Source: CAD feature listing. Evaluate the final solid. Frame: model axes, mm. A direction names the side the tool comes from. Give positions to 0.01 mm unless a question says otherwise; leave off trailing zeros. Order: outer loops, then holes, each group sorted by start corner. A loop starts at its lowest first (then second) coordinate and runs counter-clockwise, first axis right, second up.
Autodesk Inventor part; units mm, degrees
ref_plane "YZ Plane" through (0, 0, 0) normal (1, 0, 0) x (0, 1, 0)
ref_plane "XZ Plane" through (0, 0, 0) normal (0, 1, 0) x (-1, 0, 0)
ref_plane "XY Plane" through (0, 0, 0) normal (0, 0, 1) x (1, 0, 0)
sketch "Sketch1" plane through (0, 0, 0) normal (0, 0, 1) x (1, 0, 0)
  circle A0 centre (0, 0) radius 6.35
  dimension "d0" = 12.7
extrude "Extrusion1" add sketch "Sketch1" along normal blind 5.08 and the other way blind 16.02
sketch "Sketch4" plane through (0, 0, 0) normal (0, 0, 1) x (1, 0, 0)
  circle A0 centre (0, 0) radius 12.065
  dimension "d9" = 24.13
extrude "Extrusion3" add sketch "Sketch4" against normal blind 1.02
sketch "Sketch5" plane through (0, 0, 5.08) normal (0, 0, 1) x (1, 0, 0)
  circle A0 centre (0, 0) radius 6.35
  circle A1 centre (0, 0) radius 2.415
  dimension "d12" = 4.83
extrude "Extrusion4" add sketch "Sketch5" along normal blind 6.86 contours A1
sketch "Sketch6" plane through (0, 0, 0) normal (0, 0, 1) x (1, 0, 0)
  circle A0 centre (0, 0) radius 6.35
  circle A1 centre (0, 9.21) radius 1.64
  circle A2 centre (0, 0) radius 9.21 construction
  line L0 (0, 0) -> (0, 14.2117) construction
  dimension "d15" = 18.42
  dimension "d16" = 3.28
extrude "Extrusion5" cut sketch "Sketch6" against normal through all contours A1
pattern_circular "Circular Pattern1" count 3 over 360 about axis through (0, 0, -10) along (0, 0, 1) of "Extrusion5"
properties part number "Slip_Ring"
1) Section query C-C, the plane y = 0. Return the cut outline in (x, z) (3 decimals).
Report:
outline: (-12.065, -1.02) - (-6.35, -1.02) - (-6.35, -16.02) - (6.35, -16.02) - (6.35, -1.02) - (12.065, -1.02) - (12.065, 0) - (6.35, 0) - (6.35, 5.08) - (2.415, 5.08) - (2.415, 11.94) - (-2.415, 11.94) - (-2.415, 5.08) - (-6.35, 5.08) - (-6.35, 0) - (-12.065, 0) - close
2) Material intervals for L1, parallel to Y at x = 0, z = -0.6 (3 decimals); L2, parallel to Z at x = 4.25, y = -5; L3, parallel to Z at x = -0.75, y = 6.25, sorted ascending.
Report:
L1: y = -12.065 to 7.57, 10.85 to 12.065
L2: z = -1.02 to 0
L3: z = -16.02 to 5.08
3) Pin query (flat end, axial travel): pin 1 (10 mm diameter, centred on y = 0.5, z = 7.5, fed in from +X); pin 2 (8 mm diameter, centred on y = 1.5, z = 8.5, fed in from -X); pin 3 (10 mm diameter, centred on y = -6.5, z = 0.5, fed in from -X). Return the tip coordinate at first contact, or that it passes through.
Report:
pin 1: stops at x = 6.35
pin 2: stops at x = -6.35
pin 3: stops at x = -11.97
4) Section query A-A, the plane x = 0. Return the cut outline in (y, z) (3 decimals), and give its area (3 significant figures).
Report:
outline: (-12.065, -1.02) - (-6.35, -1.02) - (-6.35, -16.02) - (6.35, -16.02) - (6.35, -1.02) - (7.57, -1.02) - (7.57, 0) - (6.35, 0) - (6.35, 5.08) - (2.415, 5.08) - (2.415, 11.94) - (-2.415, 11.94) - (-2.415, 5.08) - (-6.35, 5.08) - (-6.35, 0) - (-12.065, 0) - close; (10.85, -1.02) - (12.065, -1.02) - (12.065, 0) - (10.85, 0) - close
area: 309 mm2
5) Section query D-D, the plane z = 1.25. Return the cut outline in (x, y), and give its area (3 significant figures).
Report:
outline: circle Ø12.7 at (0, 0)
area: 127 mm2
6) Reachability of faces 1 (the cylindrical face through (-0.36, 7.61, -0.5)), 2 (the flat face through (5, -5, 0)), 3 (the cylindrical face through (-1.38, -6.2, -8.41)) from +Z, -Z, +X, -X, +Y, -Y: full face, straight path, thin tool, end or side. Return the list, or none.
Report:
face 1: +Z, -Z
face 2: +Z
face 3: -Z
7) Section query B-B, the plane y = 9.21. Return the cut outline in (x, z).
Report:
outline: (-7.79, -1.02) - (-1.64, -1.02) - (-1.64, 0) - (-7.79, 0) - close; (1.64, -1.02) - (7.79, -1.02) - (7.79, 0) - (1.64, 0) - close
8) Draft query along Y for faces 4 (the cylindrical face through (-2.413, -0.106, 8.462)), 5 (the cylindrical face through (-9.185, -3.497, -0.503)), 6 (the flat face through (5, -5, -1.02)). Return one class per face: +Y half, -Y half, draft (parallel to the pull), parting line (faces both ways), or undercut.
Report:
face 4: parting line
face 5: undercut
face 6: draft
